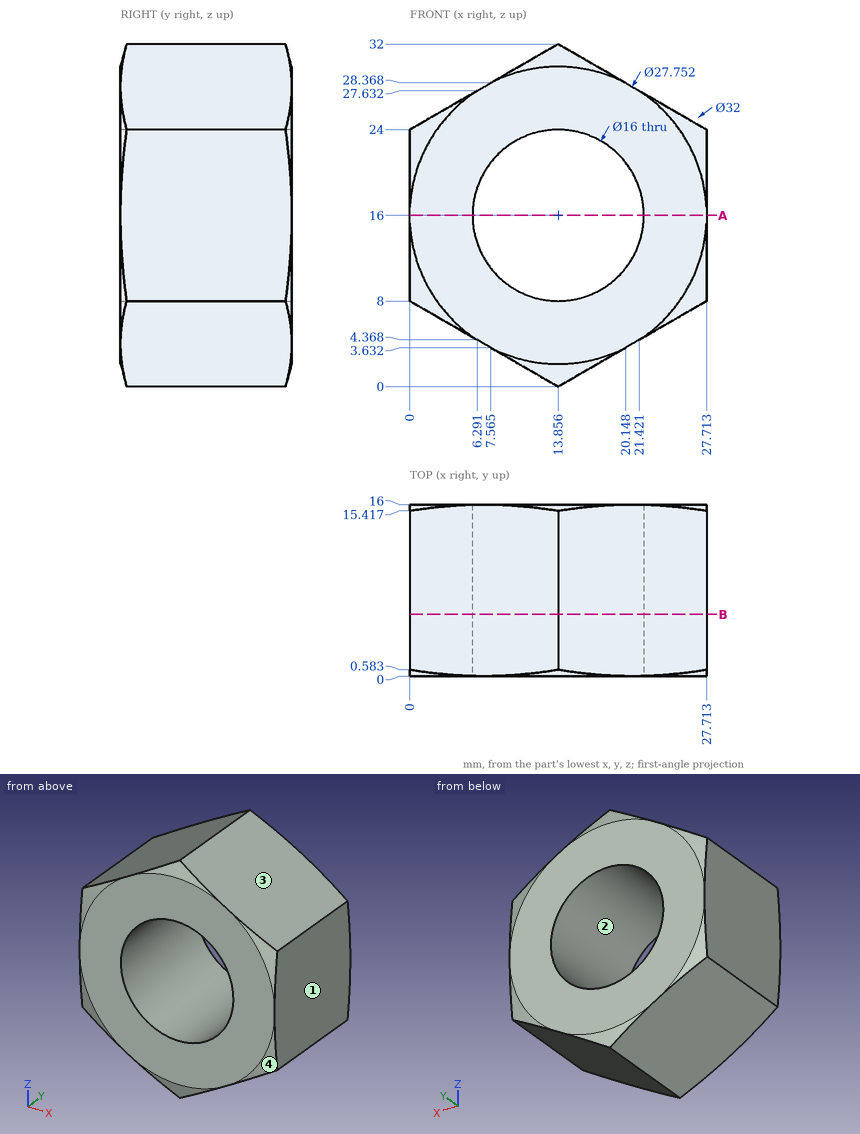
Answer from the drawing. Dimensions are ordinates in mm from the lowest x, y and z of the part. Give positions to 0.01 mm unless a question says otherwise; leave off trailing zeros. Loops run counter-clockwise (first coordinate to the right, second up) from the corner with the lowest first, then second, coordinate; pieces in that order, holes last. Notation, with made-up numbers: (29, -26.5) - (46, -26.5) arc R29 cw to (46, 0.5) - close; hole circle Ø2 at (15, 12.25). An arc over 180 degrees is marked (long way). Answer as CSV lines item,"result". Start each with the question number.
Item 1: Each of these flat-tipped pins is pushed along its axis until it touches: pin 1 (3 mm diameter, centred on x = 3, y = 4.5, fed in from -Z); pin 2 (4 mm diameter, centred on x = 10.5, y = 6.5, fed in from -Z); pin 3 (4 mm diameter, centred on x = 14, y = 9, fed in from -Z). Where does it stop, or does it pass through?
Item 2: Find the intervals of material crossed by line 1 (X direction, y = 8.5, z = 16); line 2 (Z direction, x = 12.5, y = 11) (1 decimal); line 3 (Z direction, x = 12, y = 10.75), in increasing order. Write a range as from..to.
Item 3: A cutting plane is placed at A-A on z = 16. Determine the outline of the cut face in (x, y).
Item 4: A cutting plane is placed at B-B on y = 5.75. Determine the outline of the cut face in (x, z).
Item 5: The mould has two halves that part along Z. Classify the marked faces 1, 2, 3 and 4: +Z half, -Z half, draft (parallel to the pull), parting line (faces both ways), or undercut.
Found:
1,pin 1,"stops at z = 5.4"
1,pin 2,"stops at z = 0.78"
1,pin 3,"stops at z = 0"
2,line 1,"x = 0..5.86, 21.86..27.71"
2,line 2,"z = 0.8..8.1, 23.9..31.2"
2,line 3,"z = 1.07..8.22, 23.78..30.93"
3,outline,"(0, 0) - (5.86, 0) - (5.86, 16) - (0, 16) - close; (21.86, 0) - (27.71, 0) - (27.71, 16) - (21.86, 16) - close"
4,outline,"(0, 8) - (13.86, 0) - (27.71, 8) - (27.71, 24) - (13.86, 32) - (0, 24) - close; hole circle Ø16 at (13.86, 16)"
5,face 1,"draft"
5,face 2,"undercut"
5,face 3,"+Z half"
5,face 4,"-Z half"
